from build123d import *

# Parameters (mm, degrees)
F0_W          = 13.3
F0_H          = 13.3
F0_W_2        = 10.3
F0_H_2        = 10.3
F1_DEPTH      = 20
F2_DEPTH      = 1.5
F3_W          = 4
F3_H          = 13.3
F4_DEPTH      = 13.3
F5_T1_DEPTH   = 37.3
F5_T3_DEPTH   = 37.3
F6_R          = 1.975
F7_DEPTH      = 25
F7_DEPTH_BACK = 25


# Not quite as in the source:
# - a fillet or chamfer that OpenCascade refuses, or shapes differently, is made with other operations: its cross-section is extruded or revolved along the edge and cut away or added


with BuildPart() as f1:
    # F0 (on Top) → F1 (new body)
    with BuildSketch(Plane.XY):
        Rectangle(F0_W, F0_H)
        Rectangle(F0_W_2, F0_H_2, mode=Mode.SUBTRACT)
    extrude(amount=-F1_DEPTH)

    # F0 (on Top) → F2 (join)
    with BuildSketch(Plane.XY):
        Rectangle(F0_W, F0_H)
        Rectangle(F0_W_2, F0_H_2, mode=Mode.SUBTRACT)
        Rectangle(F0_W_2, F0_H_2)
    extrude(amount=F2_DEPTH)

    # F3 (on face) → F4 (join)
    with BuildSketch(Plane.XY.offset(1.5)):
        with Locations((-4.65, 0)):
            Rectangle(F3_W, F3_H)
        with Locations((4.65, 0)):
            Rectangle(F3_W, F3_H)
    extrude(amount=F4_DEPTH)

    # F5: fillet of radius 6.66 on 4 edges, made by hand

    # F5_s2 → F5_t1 (cut)
    with BuildSketch(Plane.YZ.offset(-14)):
        with BuildLine():
            ThreePointArc((-0.01, 14.8), (4.6993311627, 12.8493311627), (6.65, 8.14))
            Line((6.65, 8.14), (6.65, 14.8))
            Line((6.65, 14.8), (-0.01, 14.8))
        make_face()
        with BuildLine():
            ThreePointArc((-6.65, 8.14), (-4.6993311627, 12.8493311627), (0.01, 14.8))
            Line((0.01, 14.8), (-6.65, 14.8))
            Line((-6.65, 14.8), (-6.65, 8.14))
        make_face()
    extrude(amount=F5_T1_DEPTH, mode=Mode.SUBTRACT)

    # F5_s4 → F5_t3 (cut)
    with BuildSketch(Plane.YZ.offset(-23.3)):
        with BuildLine():
            ThreePointArc((-0.01, 14.8), (4.6993311627, 12.8493311627), (6.65, 8.14))
            Line((6.65, 8.14), (6.65, 14.8))
            Line((6.65, 14.8), (-0.01, 14.8))
        make_face()
        with BuildLine():
            ThreePointArc((-6.65, 8.14), (-4.6993311627, 12.8493311627), (0.01, 14.8))
            Line((0.01, 14.8), (-6.65, 14.8))
            Line((-6.65, 14.8), (-6.65, 8.14))
        make_face()
    extrude(amount=F5_T3_DEPTH, mode=Mode.SUBTRACT)

    # F6 (on face) → F7 (cut, two sides)
    with BuildSketch(Plane.YZ.offset(6.65)) as f7_sk:
        with Locations((0.01, 8.14)):
            Circle(F6_R)
    extrude(amount=-F7_DEPTH, mode=Mode.SUBTRACT)
    extrude(f7_sk.sketch, amount=F7_DEPTH_BACK, mode=Mode.SUBTRACT)


solid = f1.part
For this review, take the finished solid that the model builds, in its own axes (mm). A direction names the side the tool comes from. Coordinates: 2 decimals unless noted, no trailing zeros. Write each loop counter-clockwise with the first axis right and the second up, starting at its lowest first coordinate (ties: lowest second). Pieces come first, ordered by that corner, then holes. Notation, with made-up numbers: (-12, -7.5) -> (38, -7.5) arc R14 ccw to (38, -2.5) -> close; hole circle Ø2 at (42, -11). An arc over 180 degrees is marked (long way). Write each question's results on one line, items separated by ' | '. Start each with the question number.
1) Consider section C-C (x = 4). Write out the cut boundary in (y, z) (3 decimals), plus the area to 3 significant figures.
2) Consider section B-B (x = -1.75). Write out the cut boundary in (y, z), plus the area to 4 significant figures.
3) Consider section D-D (y = 5.75). Write out the cut boundary in (x, z).
4) Insertion check: pin 1 (2 mm diameter, centred on x = -4.5, y = 1.5, fed in from +Z); pin 2 (3.5 mm diameter, centred on y = 0.01, z = 8.14, fed in from +X); pin 3 (6 mm diameter, centred on x = -2, y = -1.5, fed in from -Z); pin 4 (5 mm diameter, centred on y = 0.01, z = 8.14, fed in from -X). Each pin has a flat end and moves straight along its axis. Give the tip position at first contact, or say it passes through.
5) Consider section A-A (z = -7.5). Write out the cut boundary in (x, y), plus the area to 3 significant figures.
6) Wall thickness on L1, parallel to Y at x = 0.75, z = -2; L2, parallel to X at y = -5.5, z = 7: over which ranges is each line inside the solid? List them lowest first. Write a range as [from, to].
7) For faces 1 (the face through (0, -5.15, -10)), 2 (the face through (-2.65, -2, 7)), 3 (the face through (-4.68, 4.65, 12.9)), list the 3-axis set-ups (+Z, -Z, +X, -X, +Y, -Y) from which the entire face can be reached by the end or side of a thin tool; tool diameter is ignored.
8) The part is to be moulded in two halves that separate along Z. For faces 4 (the face through (-4.622, -0.418, 6.212)), 5 (the face through (6.65, 0, -3)), 6 (the face through (0, 0, 1.5)), say which applies: +Z half, -Z half, draft (parallel to the pull), parting line (faces both ways), or undercut.
Geometry says:
1) outline: (-6.65, -20) -> (-5.15, -20) -> (-5.15, 0) -> (5.15, 0) -> (5.15, -20) -> (6.65, -20) -> (6.65, 8.14) arc R6.66 ccw to (0, 14.8) arc R6.66 ccw to (-6.65, 8.14) -> close; hole circle Ø3.95 at (0.01, 8.14) | area: 226 mm^2
2) outline: (-6.65, -20) -> (-5.15, -20) -> (-5.15, 0) -> (5.15, 0) -> (5.15, -20) -> (6.65, -20) -> (6.65, 1.5) -> (-6.65, 1.5) -> close | area: 79.95 mm^2
3) outline: (-6.65, -20) -> (6.65, -20) -> (6.65, 11.48) -> (2.65, 11.48) -> (2.65, 1.5) -> (-2.65, 1.5) -> (-2.65, 11.48) -> (-6.65, 11.48) -> close
4) pin 1: z = 14.78 | pin 2: through | pin 3: z = 0 | pin 4: x = -6.65
5) outline: (-6.65, -6.65) -> (6.65, -6.65) -> (6.65, 6.65) -> (-6.65, 6.65) -> close; hole (-5.15, -5.15) -> (5.15, -5.15) -> (5.15, 5.15) -> (-5.15, 5.15) -> close | area: 70.8 mm^2
6) L1: [-6.65, -5.15], [5.15, 6.65] | L2: [-6.65, -2.65], [2.65, 6.65]
7) face 1: -Z | face 2: +Z, +Y, -Y | face 3: +Z, +X, -X, +Y
8) face 4: undercut | face 5: draft | face 6: +Z half
